from build123d import *

# Parameters (mm, degrees)
F1_DEPTH = 158.75
F2_R     = 4
F3_DEPTH = 12.7
F4_SIZE  = 0.762
F5_D     = 14
F5_DEPTH = 16.16
F5_TIP   = 4.2060243332


with BuildPart() as f1:
    # F0 (on Right) → F1 (new body)
    with BuildSketch(Plane.YZ):
        Polygon((0, 25.4), (0, 0), (3.175, 0), (3.175, 3.175), (130.175, 3.175), (130.175, 0), (133.35, 0), (133.35, 25.4), align=None)
    extrude(amount=F1_DEPTH)

    # F2 (on face) → F3 (cut)
    with BuildSketch(Plane.XY.offset(25.4)):
        with Locations((79.375, 95.25)):
            Circle(F2_R)
        with Locations((50.8, 66.675)):
            Circle(F2_R)
        with Locations((79.375, 38.1)):
            Circle(F2_R)
        with Locations((107.95, 66.675)):
            Circle(F2_R)
    extrude(amount=-F3_DEPTH, mode=Mode.SUBTRACT)

    # F4
    f4_edges = [f1.edges().sort_by_distance(p)[0] for p in [
        (75.375, 95.25, 25.4),
        (103.95, 66.675, 25.4),
        (75.375, 38.1, 25.4),
        (46.8, 66.675, 25.4),
        (79.375, 133.35, 25.4),
        (0, 66.675, 25.4),
        (79.375, 0, 25.4),
        (158.75, 66.675, 25.4),
    ]]
    chamfer(f4_edges, length=F4_SIZE)

    # F5
    with Locations(Plane.XY.offset(25.4)):
        with Locations((79.375, 66.675)):
            Hole(F5_D / 2, depth=F5_DEPTH)
            with Locations((0, 0, -(F5_DEPTH + F5_TIP / 2))):  # 118° drill point
                Cone(0, F5_D / 2, F5_TIP, mode=Mode.SUBTRACT)


solid = f1.part
Source: CAD feature listing. Evaluate the final solid. Frame: model axes, mm. A direction names the side the tool comes from. Round coordinates to 2 decimals unless told otherwise and drop trailing zeros. Loops run counter-clockwise (first coordinate to the right, second up) from the corner with the lowest first, then second, coordinate; pieces in that order, holes last. Notation, with made-up numbers: M 51,-37.5 L 93,-37.5 A10 ccw 93,-20.5 Z; hole C 86,16.25 d10. An arc over 180 degrees is marked long. Return JSON: item names as keys, results as strings. Group by question number.
1. Reachability of faces 1 (the face through (78, 66, 3.175)), 2 (the face through (78, 53, 25.4)), 3 (the face through (52.65, 63.13, 18.75)) from +Z, -Z, +X, -X, +Y, -Y: full face, straight path, thin tool, end or side. Return the list, or none.
2. Mould query, pull axis Y, two halves, no side actions, for faces 4 (the face through (0, 66, 12)), 5 (the face through (78, 3.175, 2)), 6 (the face through (78, 0, 12)), 7 (the face through (75.38, 38.28, 18.75)). Classes: released by +Y, released by -Y, zero draft, split by the parting line, or undercut.
3. Section query B-B on y = 95.25. Output: boundary loops of the cut face in (x, z) (3 decimals).
4. Pin query (flat end, axial travel): pin 1 (2.5 mm diameter, centred on x = 50, y = 67, fed in from +Z); pin 2 (6.5 mm diameter, centred on x = 79.375, y = 38.1, fed in from -Z) (3 decimals); pin 3 (4 mm diameter, centred on x = 107, y = 68.5, fed in from +Z). Return the tip coordinate at first contact, or that it passes through.
5. Section query C-C on z = 21.25. Output: boundary loops of the cut face in (x, y) (3 decimals), and give its area (3 significant figures).
6. Section query D-D on y = 58. Output: boundary loops of the cut face in (x, z) (3 decimals), and give its area (3 significant figures).
7. Material intervals for line 1 along Y through (x, z) = (107.95, 20.5) (3 decimals); line 2 along Y through (x, z) = (87, 2.75) (3 decimals); line 3 along Z through (x, y) = (94, 29) (3 decimals), sorted ascending. Write a range as from..to.
8. Section query A-A on x = 50.8. Output: boundary loops of the cut face in (y, z) (3 decimals).
Checks:
{
 "1": {"face 1": "-Z, +X, -X", "face 2": "+Z, +X, -X, +Y, -Y", "face 3": "+Z"},
 "2": {"face 4": "zero draft", "face 5": "undercut", "face 6": "released by -Y", "face 7": "undercut"},
 "3": {"outline": "M 0,3.175 L 158.75,3.175 L 158.75,24.638 L 157.988,25.4 L 84.137,25.4 L 83.375,24.638 L 83.375,12.7 L 75.375,12.7 L 75.375,24.638 L 74.613,25.4 L 0.762,25.4 L 0,24.638 Z"},
 "4": {"pin 1": "stops at z = 12.7", "pin 2": "stops at z = 3.175", "pin 3": "stops at z = 24.7"},
 "5": {"outline": "M 0,0 L 158.75,0 L 158.75,133.35 L 0,133.35 Z; hole C 50.8,66.675 d8; hole C 79.375,66.675 d14; hole C 79.375,38.1 d8; hole C 79.375,95.25 d8; hole C 107.95,66.675 d8", "area": "20,800 mm²"},
 "6": {"outline": "M 0,3.175 L 158.75,3.175 L 158.75,24.638 L 157.988,25.4 L 0.762,25.4 L 0,24.638 Z", "area": "3,530 mm²"},
 "7": {"line 1": "y = 0..62.675, 70.675..133.35", "line 2": "y = 0..3.175, 130.175..133.35", "line 3": "z = 3.175..25.4"},
 "8": {"outline": "M 0,0 L 3.175,0 L 3.175,3.175 L 130.175,3.175 L 130.175,0 L 133.35,0 L 133.35,24.638 L 132.588,25.4 L 71.437,25.4 L 70.675,24.638 L 70.675,12.7 L 62.675,12.7 L 62.675,24.638 L 61.913,25.4 L 0.762,25.4 L 0,24.638 Z"}
}
